CAD build for the part. Positions are in the model's coordinates, mm. Face numbers are marked on the shaded views. A direction names the side the tool comes from. Coordinates: 2 decimals unless noted, no trailing zeros. Write each loop counter-clockwise with the first axis right and the second up, starting at its lowest first coordinate (ties: lowest second). Pieces come first, ordered by that corner, then holes. Notation, with made-up numbers: M 78.5,88.5 L 88.5,88.5 A30 cw 88.5,119.5 Z; hole C 86.25,89.5 d6. An arc over 180 degrees is marked long. Put each result on its own line as item: value. Start each with the question number.
```python
from build123d import *

# Parameters (mm, degrees)
SM_BASE_FLANGE_1_DEPTH = 15
CUT_EXTRUDE_1_REACH    = 28.926
SKETCH_3_R             = 3.5
FILLET_1_R             = 5


# Sheet-metal steps are written as plain solids
with BuildPart() as part:
    # Sketch 1 → 基体-法兰1 (new, symmetric)
    with BuildSketch(Plane.XY):
        with BuildLine():
            Line((0, 20), (0, 2.5))
            ThreePointArc((0, 2.5), (0.732233047, 0.732233047), (2.5, 0))
            Line((2.5, 0), (12, 0))
            Line((12, 0), (12, 2))
            Line((12, 2), (2.5, 2))
            ThreePointArc((2.5, 2), (2.146446609, 2.146446609), (2, 2.5))
            Line((2, 2.5), (2, 20))
            Line((2, 20), (0, 20))
        make_face()
    extrude(amount=SM_BASE_FLANGE_1_DEPTH, both=True)

    # 草图3 → 切除-拉伸1 (cut, up to next)
    with BuildSketch(Plane(origin=(2, 0, 0), x_dir=(0, 0, -1), z_dir=(1, 0, 0)), mode=Mode.PRIVATE) as cut_extrude_1_sk1:
        with Locations(Location((-7.5, 13, 0), (0, 0, 90))):
            Circle(SKETCH_3_R)
    cut_extrude_1_tool1 = extrude(cut_extrude_1_sk1.sketch, amount=-CUT_EXTRUDE_1_REACH, mode=Mode.PRIVATE) & part.part
    # 草图3 → 切除-拉伸1 (cut, up to next)
    with BuildSketch(Plane(origin=(2, 0, 0), x_dir=(0, 0, -1), z_dir=(1, 0, 0)), mode=Mode.PRIVATE) as cut_extrude_1_sk2:
        with Locations(Location((7.5, 13, 0), (0, 0, 90))):
            Circle(SKETCH_3_R)
    cut_extrude_1_tool2 = extrude(cut_extrude_1_sk2.sketch, amount=-CUT_EXTRUDE_1_REACH, mode=Mode.PRIVATE) & part.part
    add(cut_extrude_1_tool1.solids().sort_by_distance((2, 13, 7.5))[0], mode=Mode.SUBTRACT)
    add(cut_extrude_1_tool2.solids().sort_by_distance((2, 13, -7.5))[0], mode=Mode.SUBTRACT)

    # 圆角1
    fillet_1_edges = [part.edges().sort_by_distance(p)[0] for p in [
        (1, 20, -15),
        (12, 1, -15),
        (1, 20, 15),
        (12, 1, 15),
    ]]
    fillet(fillet_1_edges, radius=FILLET_1_R)


solid = part.part
```
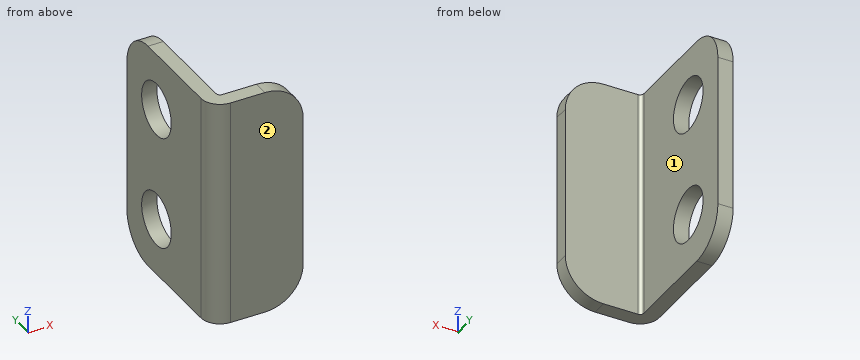
(1) Slice it at C-C, the plane z = -13. Write the cut outline in (x, y).
(2) Slice it at A-A, the plane y = 13. Write the cut outline in (x, z), then the cut area to 3 significant figures.
(3) Which spindle directions (+Z, -Z, +X, -X, +Y, -Y) get a long thin tool onto all of the face, cutting with end or side? Do the marked faces 1 and 2. Say none if no direction does.
(4) Drop flat-ended pins along their axis: pin 1 (9 mm diameter, centred on y = 13.5, z = 4, fed in from +X); pin 2 (2 mm diameter, centred on x = 10.5, z = -10.5, fed in from -Y); pin 3 (5 mm diameter, centred on x = 8.5, z = 6, fed in from +Y). Give the stop position or say it passes through.
(5) Slice it at B-B, the plane z = 7.5. Write the cut outline in (x, y), then the cut area to 3 significant figures.
(6) Slice it at D-D, the plane y = 16. Write the cut outline in (x, z), then the cut area to 3 significant figures.
(7) Drill centre lines: line 1 (Z direction, x = 1.4, y = 13); line 2 (Z direction, x = 1.75, y = 15.5); line 3 (X direction, y = 6, z = -10). Where is each one in solid material? Low to high. Write a range as [from, to].
Result set:
1. outline: M 0,2.5 A2.5 ccw 2.5,0 L 11,0 L 11,2 L 2.5,2 A0.5 cw 2,2.5 L 2,19 L 0,19 Z
2. outline: M 0,-15 L 2,-15 L 2,-11 L 0,-11 Z; M 0,-4 L 2,-4 L 2,4 L 0,4 Z; M 0,11 L 2,11 L 2,15 L 0,15 Z
2. area: 32.0 mm^2
3. face 1: +Z, -Z, +X, +Y
3. face 2: +Z, -Z, +X, -X, -Y
4. pin 1: stops at x = 2
4. pin 2: stops at y = 0
4. pin 3: stops at y = 2
5. outline: M 0,2.5 A2.5 ccw 2.5,0 L 12,0 L 12,2 L 2.5,2 A0.5 cw 2,2.5 L 2,9.5 L 0,9.5 Z; M 0,16.5 L 2,16.5 L 2,20 L 0,20 Z
5. area: 44.7 mm^2
6. outline: M 0,-14.9 L 2,-14.9 L 2,-9.3 L 0,-9.3 Z; M 0,-5.7 L 2,-5.7 L 2,5.7 L 0,5.7 Z; M 0,9.3 L 2,9.3 L 2,14.9 L 0,14.9 Z
6. area: 45.2 mm^2
7. line 1: z = [-15, -11], [-4, 4], [11, 15]
7. line 2: z = [-14.97, -9.95], [-5.05, 5.05], [9.95, 14.97]
7. line 3: x = [0, 2]
